from build123d import *

# Parameters (mm, degrees)
SKETCH_W        = 79.03
SKETCH_H        = 156.85
PAD_DEPTH       = 14
POCKET_DEPTH    = 11.6
PAD001_DEPTH    = 10
SKETCH003_R     = 1.45
POCKET001_DEPTH = 12
FILLET_R        = 5
CHAMFER_SIZE    = 1
FILLET001_R     = 2
CHAMFER001_SIZE = 0.8
SKETCH004_W     = 12.65
SKETCH004_H     = 11
POCKET002_DEPTH = 8.6
SKETCH005_W     = 11.08
SKETCH005_H     = 10
POCKET003_DEPTH = 7
SKETCH006_R     = 1.45
POCKET004_DEPTH = 12
SKETCH007_W     = 92.15
SKETCH007_H     = 16.7
POCKET005_DEPTH = 1.6
CHAMFER002_SIZE = 0.8
CHAMFER003_SIZE = 3
CHAMFER004_SIZE = 1
POCKET006_DEPTH = 509.235242
SKETCH009_R     = 2.2
POCKET007_DEPTH = 2.2
CHAMFER005_SIZE = 0.5


with BuildPart() as part:
    # Sketch → Pad (new body)
    with BuildSketch(Plane.XY):
        with Locations((0, -69.725)):
            Rectangle(SKETCH_W, SKETCH_H)
    extrude(amount=PAD_DEPTH)

    # Sketch001 (on Face6 of Pad) → Pocket (cut)
    with BuildSketch(Plane.XY.offset(14)):
        Polygon((-37.015, -145.15), (37.015, -145.15), (37.015, 0), (27.7, 0), (27.7, 8.7), (-27.7, 8.7), (-27.7, 0), (-37.015, 0), align=None)
    extrude(amount=-POCKET_DEPTH, mode=Mode.SUBTRACT)

    # Sketch002 (on Face6 of Pocket) → Pad001 (join)
    with BuildSketch(Plane.XY.offset(2.4)):
        Polygon((-35.015, 0), (-35.015, -7.5), (-34.015, -8.5), (-34.015, -135.15), (-27.015, -142.15), (27.015, -142.15), (34.015, -135.15), (34.015, -8.5), (35.015, -7.5), (35.015, 0), (37.015, 0), (37.015, -145.15), (-37.015, -145.15), (-37.015, 0), align=None)
    extrude(amount=PAD001_DEPTH)

    # Sketch003 (on Face24 of Pad001) → Pocket001 (cut)
    with BuildSketch(Plane.XY.offset(12.4)):
        with Locations((-33.34, -141.47)):
            Circle(SKETCH003_R)
        with Locations((33.34, -141.47)):
            Circle(SKETCH003_R)
    extrude(amount=-POCKET001_DEPTH, mode=Mode.SUBTRACT)

    # Fillet
    fillet_edges = [part.edges().sort_by_distance(p)[0] for p in [
        (39.515, 8.7, 7),
        (39.515, -148.15, 7),
        (-39.515, 8.7, 7),
        (-39.515, -148.15, 7),
    ]]
    fillet(fillet_edges, radius=FILLET_R)

    # Chamfer
    chamfer_edges = [part.edges().sort_by_distance(p)[0] for p in [
        (-38.050534, 7.235534, 0),
    ]]
    chamfer(chamfer_edges, length=CHAMFER_SIZE)

    # Fillet001
    fillet001_edges = [part.edges().sort_by_distance(p)[0] for p in [
        (-38.050534, 7.235534, 1),
    ]]
    fillet(fillet001_edges, radius=FILLET001_R)

    # Chamfer001
    chamfer001_edges = [part.edges().sort_by_distance(p)[0] for p in [
        (-34.79, -141.47, 12.4),
        (31.89, -141.47, 12.4),
    ]]
    chamfer(chamfer001_edges, length=CHAMFER001_SIZE)

    # Sketch004 (on Face20 of Chamfer001) → Pocket002 (cut)
    with BuildSketch(Plane.XY.offset(14)):
        with Locations((37.485, -27.31)):
            Rectangle(SKETCH004_W, SKETCH004_H)
    extrude(amount=-POCKET002_DEPTH, mode=Mode.SUBTRACT)

    # Sketch005 (on Face16 of Pocket002) → Pocket003 (cut)
    with BuildSketch(Plane.XY.offset(14)):
        with Locations((-36.33, -13.2)):
            Rectangle(SKETCH005_W, SKETCH005_H)
    extrude(amount=-POCKET003_DEPTH, mode=Mode.SUBTRACT)

    # Sketch006 → Pocket004 (cut)
    with BuildSketch(Plane.XY.offset(14)):
        with Locations((-33.34, 3.5)):
            Circle(SKETCH006_R)
        with Locations((33.34, 3.5)):
            Circle(SKETCH006_R)
    extrude(amount=-POCKET004_DEPTH, mode=Mode.SUBTRACT)

    # Sketch007 (on Face7 of Pocket004) → Pocket005 (cut)
    with BuildSketch(Plane.XY.offset(14)):
        with Locations((0, 8.35)):
            Rectangle(SKETCH007_W, SKETCH007_H)
    extrude(amount=-POCKET005_DEPTH, mode=Mode.SUBTRACT)

    # Chamfer002
    chamfer002_edges = [part.edges().sort_by_distance(p)[0] for p in [
        (31.89, 3.5, 12.4),
        (-34.79, 3.5, 12.4),
    ]]
    chamfer(chamfer002_edges, length=CHAMFER002_SIZE)

    # Chamfer003
    chamfer003_edges = [part.edges().sort_by_distance(p)[0] for p in [
        (-39.515, -8.2, 10.5),
        (-39.515, -13.2, 7),
        (-39.515, -18.2, 10.5),
    ]]
    chamfer(chamfer003_edges, length=CHAMFER003_SIZE)

    # Chamfer004
    chamfer004_edges = [part.edges().sort_by_distance(p)[0] for p in [
        (39.515, -21.81, 9.7),
        (39.515, -27.31, 5.4),
        (39.515, -32.81, 9.7),
    ]]
    chamfer(chamfer004_edges, length=CHAMFER004_SIZE)

    # Sketch008 (on Face9 of Chamfer004) → Pocket006 (cut, through all)
    with BuildSketch(Plane.XZ.offset(148.15)):
        Polygon((-43, 12), (-43, 2), (-38, 7), align=None)
    pocket006 = extrude(amount=-POCKET006_DEPTH, mode=Mode.SUBTRACT)

    # Mirrored: Pocket006 across Sketch008 V_Axis
    add(pocket006.mirror(Plane(origin=(0, -148.15, 0), x_dir=(0, -1, 0), z_dir=(1, 0, 0))), mode=Mode.SUBTRACT)

    # Sketch009 (on Face56 of Mirrored) → Pocket007 (cut)
    with BuildSketch(Plane(origin=(0, 8.7, 0), x_dir=(-1, 0, 0), z_dir=(0, 1, 0))):
        with Locations((-31, 7)):
            Circle(SKETCH009_R)
    pocket007 = extrude(amount=-POCKET007_DEPTH, mode=Mode.SUBTRACT)

    # Mirrored001: Pocket007 across Sketch009 V_Axis
    add(pocket007.mirror(Plane(origin=(0, 8.7, 0), x_dir=(0, 1, 0), z_dir=(-1, 0, 0))), mode=Mode.SUBTRACT)

    # Chamfer005
    chamfer005_edges = [part.edges().sort_by_distance(p)[0] for p in [
        (33.2, 8.7, 7),
        (-33.2, 8.7, 7),
    ]]
    chamfer(chamfer005_edges, length=CHAMFER005_SIZE)


solid = part.part
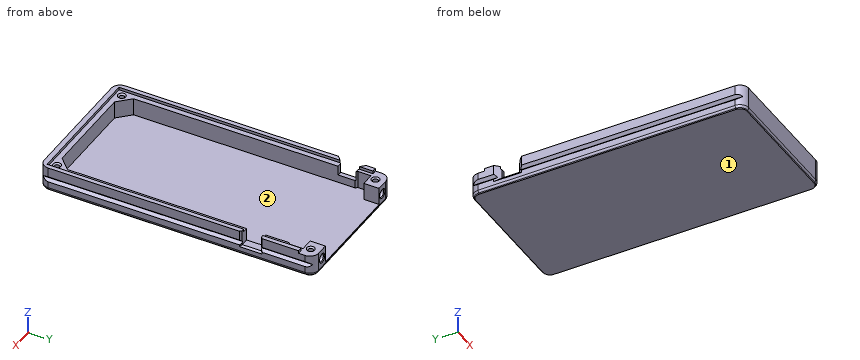
Read the model definition and answer for the solid it produces. Units are mm, in the model's axes. Face numbers are marked on the shaded views. Coordinates: 2 decimals unless noted, no trailing zeros. Loops run counter-clockwise (first coordinate to the right, second up) from the corner with the lowest first, then second, coordinate; pieces in that order, holes last.
Q1. The mould has two halves that part along X. Classify the marked faces 1 and 2: +X half, -X half, draft (parallel to the pull), parting line (faces both ways), or undercut.
Q2. The part is cut by section B-B on x = -20. Write down the section's boundary in (y, z).
Q3. Each of these flat-tipped pins is pushed along its axis until it touches: pin 1 Ø1.3 at (x, z) = (36.5, 10.5) entering from +Y; pin 2 Ø5 at (x, y) = (37, -25) entering from +Z; pin 3 Ø1.2 at (x, z) = (-35.5, 9.5) entering from +Y; pin 4 Ø13 at (x, y) = (36.5, -2.5) entering from +Z. Where does it stop, or does it pass through?
Q4. Consider probe 1 along X at (y, z) = (-141.47, 7.5) (3 decimals); probe 2 along Z at (x, y) = (31, 7); probe 3 along X at (y, z) = (-58.5, 13.75) (3 decimals). Determine where each line is inside the solid, lowest interval first.
Q5. The part is cut by section C-C on y = -30.5. Write down the section's boundary in (x, z) (3 decimals), and give its area (3 significant figures).
Q6. The part is cut by section A-A on y = -76.5. Write down the section's boundary in (x, z) (3 decimals), and give its area (3 significant figures).
Results below:
1. face 1: draft
1. face 2: undercut
2. outline: (-148.15, 1.83) arc R2 ccw to (-147.56, 0.41) - (-147.15, 0) - (7.7, 0) - (8.11, 0.41) arc R2 ccw to (8.7, 1.83) - (8.7, 2.4) - (-142.15, 2.4) - (-142.15, 12.4) - (-145.15, 12.4) - (-145.15, 14) - (-148.15, 14) - close
3. pin 1: stops at y = 8.52
3. pin 2: stops at z = 5.4
3. pin 3: stops at y = 8.69
3. pin 4: stops at z = 14
4. probe 1: x = -38.5 to -34.79, -31.89 to -27.695, 27.695 to 31.89, 34.79 to 38.5
4. probe 2: z = 0 to 4.8, 9.2 to 12.4
4. probe 3: x = -39.515 to -37.015, 37.015 to 39.515
5. outline: (-39.515, 1.828) arc R2 ccw to (-38.929, 0.414) - (-38.515, 0) - (38.515, 0) - (38.929, 0.414) arc R2 ccw to (39.515, 1.828) - (39.515, 4.4) - (38.515, 5.4) - (34.015, 5.4) - (34.015, 2.4) - (-34.015, 2.4) - (-34.015, 12.4) - (-37.015, 12.4) - (-37.015, 14) - (-39.515, 14) - (-39.515, 8.515) - (-38, 7) - (-39.515, 5.485) - close
5. area: 261 mm2
6. outline: (-39.515, 1.828) arc R2 ccw to (-38.929, 0.414) - (-38.515, 0) - (38.515, 0) - (38.929, 0.414) arc R2 ccw to (39.515, 1.828) - (39.515, 5.485) - (38, 7) - (39.515, 8.515) - (39.515, 14) - (37.015, 14) - (37.015, 12.4) - (34.015, 12.4) - (34.015, 2.4) - (-34.015, 2.4) - (-34.015, 12.4) - (-37.015, 12.4) - (-37.015, 14) - (-39.515, 14) - (-39.515, 8.515) - (-38, 7) - (-39.515, 5.485) - close
6. area: 302 mm2
